Geometry check sheet. Reference: the model listing, model coordinates, mm. Face numbers are marked on the shaded views. A direction names the side the tool comes from. Round coordinates to 2 decimals unless told otherwise and drop trailing zeros. Order: outer loops, then holes, each group sorted by start corner. A loop starts at its lowest first (then second) coordinate and runs counter-clockwise, first axis right, second up. Notation, with made-up numbers: (16, 76) - (41, 76) arc R16 ccw to (41, 105) - close; hole circle Ø4 at (11.5, 82). An arc over 180 degrees is marked (long way). Return JSON: item names as keys, results as strings. Group by question number.
Q1. Sectioned sample at B-B, the plane z = 8.5. Record the cut outline in (x, y).
Q2. Sectioned sample at D-D, the plane x = -20. Record the cut outline in (y, z), then the cut area to 3 significant figures.
Q3. Sectioned sample at C-C, the plane z = -63. Record the cut outline in (x, y), then the cut area to 3 significant figures.
Q4. Draft check along X on the marked faces 1, 2, 3 and 4. Enter one of: pulls with the +X half, pulls with the -X half, needs draft (parallel to the pull), parting line crosses it, or undercut.
Q5. Gauge pin test, flat ends, axial feed: pin 1 Ø24 at (x, y) = (-119.5, -46.5) entering from -Z; pin 2 Ø4 at (x, y) = (35.5, -51) entering from -Z; pin 3 Ø3 at (y, z) = (-49, -75) entering from -X. Record the tip position at first contact, or that the pin passes through.
Q6. Sectioned sample at A-A, the plane y = -50. Record the cut outline in (x, z).
Q7. Material ranges on line 1 along Y through (x, z) = (-97, 5.5); line 2 along X through (y, z) = (-60.5, 30.5); line 3 along X through (y, z) = (-43.5, 22.5), recorded low to high.
Q8. Tool access check on the marked faces 5 and 6. Record the directions out of +Z, -Z, +X, -X, +Y, -Y that give a thin tool (end or side, any length) a straight path to the whole face; none if there is none.
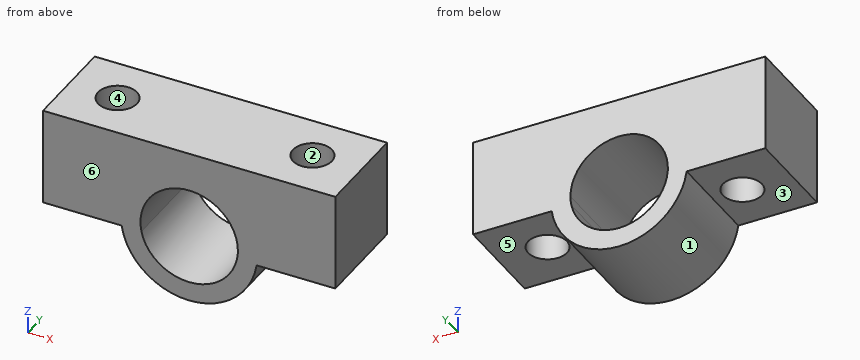
```python
from build123d import *

# Parameters (mm, degrees)
F1_DEPTH = 100
F3_D     = 40


with BuildPart() as f1:
    # F0 (on Front) → F1 (new body)
    with BuildSketch(Plane.XZ):
        with BuildLine():
            Line((151.65843, 56.57242), (-148.34157, 56.57242))
            Line((-148.34157, 56.57242), (-148.34157, -43.42758))
            Line((-148.34157, -43.42758), (-67.623602, -43.42758))
            ThreePointArc((-67.623602, -43.42758), (1.65843, -103.42758), (70.940463, -43.42758))
            Line((70.940463, -43.42758), (151.65843, -43.42758))
            Line((151.65843, -43.42758), (151.65843, 56.57242))
        make_face()
        with BuildLine():
            ThreePointArc((-47.331365, -43.42758), (-3.367018, 16.319228), (51.65843, -33.42758))
            ThreePointArc((51.65843, -33.42758), (51.405238, -38.453028), (50.648225, -43.42758))
            ThreePointArc((50.648225, -43.42758), (1.65843, -83.42758), (-47.331365, -43.42758))
        make_face(mode=Mode.SUBTRACT)
    extrude(amount=F1_DEPTH)

    # F3 (through all)
    with Locations(Plane.XY.offset(56.57242)):
        with Locations((-98.34157, -50), (101.65843, -50)):
            Hole(F3_D / 2)


solid = f1.part
```
Reply:
{
 "1": {"outline": "(-148.34, -100) - (-25.58, -100) - (-25.58, 0) - (-148.34, 0) - close; (28.9, -100) - (151.66, -100) - (151.66, 0) - (28.9, 0) - close; hole circle Ø40 at (-98.34, -50); hole circle Ø40 at (101.66, -50)"},
 "2": {"outline": "(-100, -99.99) - (0, -99.99) - (0, -78.49) - (-100, -78.49) - close; (-100, 11.64) - (0, 11.64) - (0, 56.57) - (-100, 56.57) - close", "area": "6,640 mm^2"},
 "3": {"outline": "(-61.79, -100) - (-38.66, -100) - (-38.66, 0) - (-61.79, 0) - close; (41.98, -100) - (65.11, -100) - (65.11, 0) - (41.98, 0) - close", "area": "4,630 mm^2"},
 "4": {"face 1": "parting line crosses it", "face 2": "undercut", "face 3": "needs draft", "face 4": "undercut"},
 "5": {"pin 1": "z = -43.43", "pin 2": "z = -95.77", "pin 3": "x = -55.74"},
 "6": {"outline": "(-148.34, -43.43) - (-118.34, -43.43) - (-118.34, 56.57) - (-148.34, 56.57) - close; (-78.34, -43.43) - (-67.62, -43.43) arc R70 ccw to (70.94, -43.43) - (81.66, -43.43) - (81.66, 56.57) - (-78.34, 56.57) - close; (121.66, -43.43) - (151.66, -43.43) - (151.66, 56.57) - (121.66, 56.57) - close; hole (50.65, -43.43) arc R50 ccw to (51.66, -33.43) arc R50 ccw (long way) to start"},
 "7": {"line 1": "-100 to -69.95, -30.05 to 0", "line 2": "-148.34 to -115.36, -81.32 to 84.64, 118.68 to 151.66", "line 3": "-148.34 to -117.26, -79.43 to 82.74, 120.57 to 151.66"},
 "8": {"face 5": "-Z, +X, +Y, -Y", "face 6": "+Z, -Z, +X, -X, -Y"}
}
